Autodesk Inventor part; units mm, degrees
ref_plane "YZ Plane" through (0, 0, 0) normal (1, 0, 0) x (0, 1, 0)
ref_plane "XZ Plane" through (0, 0, 0) normal (0, 1, 0) x (-1, 0, 0)
ref_plane "XY Plane" through (0, 0, 0) normal (0, 0, 1) x (1, 0, 0)
sketch "Sketch1" plane through (0, 0, 0) normal (1, 0, 0) x (0, 1, 0)
  line L0 (0, 0) -> (350, 0)
  line L1 (350, 0) -> (350, -1600)
  line L2 (350, -1600) -> (0, -1600)
  line L3 (0, -1600) -> (0, 0)
  dimension "d0" = 350
  dimension "d1" = 1600
extrude "Extrusion1" add sketch "Sketch1" along normal blind 20
sketch "Sketch3" plane through (0, 0, 0) normal (0, 0, 1) x (1, 0, 0)
  point P0 (0, 0)
sketch "Sketch6" plane through (20, 0, 0) normal (1, 0, 0) x (0, 0, -1)
  line L0 (0, 350) -> (0, 0)
  line L1 (1600, 0) -> (1600, 350)
  line L2 (0, 175) -> (1600, 175)
  line L3 (1600, 175) -> (1600, 155)
  line L4 (1600, 155) -> (0, 155)
  line L5 (0, 155) -> (0, 175)
  point P0 (0, 155)
  dimension "d11" = 20
extrude "Extrusion4" add sketch "Sketch6" along normal blind 80
sketch "Sketch7" plane through (0, 0, 0) normal (0, 0, 1) x (1, 0, 0)
  line L0 (100, 155) -> (100, 175)
  line L1 (100, 175) -> (64.6447, 210.3553)
  line L2 (100, 175) -> (150, 175) construction
  line L3 (64.6447, 210.3553) -> (29.2893, 175)
  line L4 (29.2893, 175) -> (33.532, 175)
  line L5 (20, 175) -> (100, 175)
  line L6 (33.532, 175) -> (64.6447, 206.1127)
  line L7 (64.6447, 206.1127) -> (95.7574, 175)
  point P0 (0, 0)
  dimension "d14" = 50
  dimension "d15" = 135
  dimension "d16" = 50
  dimension "d18" = 3
  dimension "d19" = 3
extrude "Extrusion5" add sketch "Sketch7" against normal blind 1600 contours L5 L7 L6 L4 L3 L1
properties part number "Riel superior"
Model file for the job. Use its own axes, mm. A direction names the side the tool comes from. Coordinates: 2 decimals unless noted, no trailing zeros. Loops run counter-clockwise (first coordinate to the right, second up) from the corner with the lowest first, then second, coordinate; pieces in that order, holes last. Notation, with made-up numbers: (-24, -11) - (16, -11) arc R8 cw to (16, -3) - close; hole circle Ø3 at (-32.5, 18). An arc over 180 degrees is marked (long way). Answer as a JSON object with one key per item and string values. Group by question number.
(1) Probe line 1 along X through (y, z) = (327, -1286.5); line 2 along Y through (x, z) = (58, -186); line 3 along Y through (x, z) = (84.5, -880). List the from-to ranges inside material, lowest first.
(2) Tool access for faces 4 (the face through (0, 173, -789)), 5 (the face through (20, 261, -789)), 6 (the face through (59, 155, -811)): list every direction of +Z, -Z, +X, -X, +Y, -Y with a clear straight run to the whole face (end or side of a thin tool).
(3) Flat gauge pins, fed straight in: pin 1 (3 mm diameter, centred on x = 23.5, z = -753, fed in from +Y); pin 2 (10 mm diameter, centred on y = 187, z = -1335, fed in from +X); pin 3 (10 mm diameter, centred on y = 219, z = -1247.5, fed in from +X). Where does each tip first touch, or does it go through?
(4) Cut at B-B (y = 42). Give the cut face in (x, z), then the cut area to 3 significant figures.
(5) Two-plate mould, pull along Y, no slides. Class faces 1 (the face through (48.87, 190.34, -788.8)), 2 (the face through (20, 76, -789)), 3 (the face through (47.214, 192.925, -788.8)): released by +Y, released by -Y, zero draft, split by the parting line, or undercut.
(6) Cut at A-A (z = -673). Give the cut face in (x, y), then the cut area to 3 significant figures.
Geometry says:
{
 "1": {"line 1": "x = 0 to 20", "line 2": "y = 155 to 175, 199.47 to 203.71", "line 3": "y = 155 to 175, 186.26 to 190.5"},
 "2": {"face 4": "+Z, -Z, -X, +Y, -Y", "face 5": "+Z, -Z, +Y", "face 6": "+Z, -Z, +X, -Y"},
 "3": {"pin 1": "stops at y = 175", "pin 2": "stops at x = 93", "pin 3": "stops at x = 20"},
 "4": {"outline": "(0, -1600) - (20, -1600) - (20, 0) - (0, 0) - close", "area": "32,000 mm^2"},
 "5": {"face 1": "undercut", "face 2": "zero draft", "face 3": "released by +Y"},
 "6": {"outline": "(0, 0) - (20, 0) - (20, 155) - (100, 155) - (100, 175) - (64.64, 210.36) - (29.29, 175) - (20, 175) - (20, 350) - (0, 350) - close; hole (33.53, 175) - (95.76, 175) - (64.64, 206.11) - close", "area": "8,880 mm^2"}
}
